Autodesk Inventor part; units mm, degrees
ref_plane "Arbeitsebene1" through (5, -117, 0) normal (0, 1, 0) x (1, 0, 0)
ref_plane "YZ Plane" through (0, 0, 0) normal (1, 0, 0) x (0, 1, 0)
ref_plane "XZ Plane" through (0, 0, 0) normal (0, 1, 0) x (-1, 0, 0)
sketch "Skizze1" plane through (0, 0, 0) normal (0, 0, 1) x (1, 0, 0)
  line L0 (0, 0) -> (60, 0)
  line L1 (60, 0) -> (60, -150)
  line L2 (60, -150) -> (0, -150)
  line L3 (0, -150) -> (0, 0)
  circle A0 centre (30, -117) radius 9
  dimension "d0" = 60
  dimension "d1" = 150
  dimension "d2" = 18
extrude "Extrusion1" add sketch "Skizze1" along normal blind 10
sketch "Skizze2" plane through (0, -150, 0) normal (0, -1, 0) x (1, 0, 0)
  point P0 (0, 0)
  point P1 (6.5, 5)
  point P2 (53.5, 5)
sketch "Skizze3" plane through (0, 0, 0) normal (0, 0, -1) x (-1, 0, 0)
  line L0 (-5, -117) -> (-55, -117)
  point P0 (0, 0)
ref_plane "Arbeitsebene1" through (5, -117, 0) normal (0, 1, 0) x (1, 0, 0)
split "Trennen1" plane through (5, -117, 0) removes the side toward (0, 1, 0)
hole "Bohrung2" at (6.5, -150, 5) at (53.5, -150, 5) direction (0, 1, 0) diameter 6.6 end through all
properties part number "Steher oben Rohr"
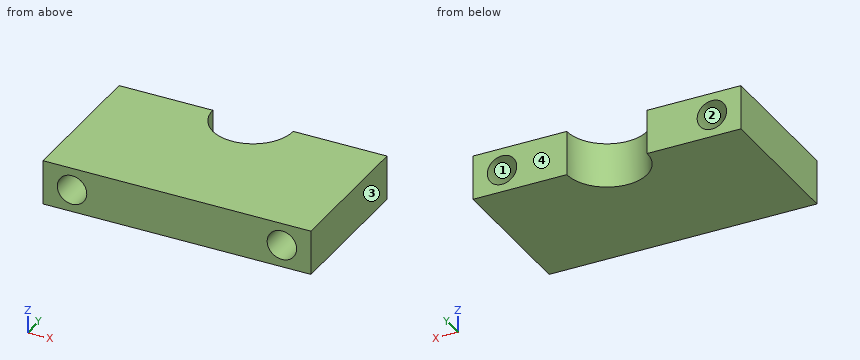
Can you work these out from the model? Positions are in its coordinate system, mm. Face numbers are marked on the shaded views. Round coordinates to 2 decimals unless told otherwise and drop trailing zeros. Loops run counter-clockwise (first coordinate to the right, second up) from the corner with the lowest first, then second, coordinate; pieces in that order, holes last. Notation, with made-up numbers: (-22, 78.5) - (-18, 78.5) arc R10 cw to (-18, 93.5) - close; hole circle Ø11 at (1.25, 13). An arc over 180 degrees is marked (long way). Write item = value, one per line. Start each with the question number.
(1) If we section it at B-B (x = 6.5): Please give me the cut outline in (y, z), and give its area (3 significant figures).
(2) If I drill on probe 1 along X at (y, z) = (-136.5, 5); probe 2 along Z at (x, y) = (6.5, -137.5); probe 3 along X at (y, z) = (-138.5, 2.75), over which ranges is the centre line in solid material (lowest first)? Write a range as [from, to].
(3) If we mould it in two halves opening along X, with no side actions, what happens to the marked faces 1, 2, 3 and 4? For each: released by +X, released by -X, zero draft, split by the parting line, or undercut.
(4) If we section it at D-D (y = -140.5): Please give me the cut outline in (x, z).
(5) If we section it at C-C (y = -125): Please give me the cut outline in (x, z), and give its area (3 significant figures).
(6) If we section it at A-A (z = 5): Please give me the cut outline in (x, y).
(7) For P1, Ø4, axis at x = 27.5, z = 9, coming from the +Y side; P2, Ø6, axis at x = 19, y = -145.5, coming from the -Z side; P3, Ø4, axis at x = 53.5, z = 5, coming from the +Y side, each with a flat end and sliding along its axis, tell me the tip position at first contact or that it passes through.
Ans:
q1.outline = (-150, 0) - (-117, 0) - (-117, 1.7) - (-150, 1.7) - close; (-150, 8.3) - (-117, 8.3) - (-117, 10) - (-150, 10) - close
q1.area = 112 mm²
q2.probe_1 = [0, 3.2], [9.8, 50.2], [56.8, 60]
q2.probe_2 = [0, 1.7], [8.3, 10]
q2.probe_3 = [0, 4.09], [8.91, 51.09], [55.91, 60]
q3.face_1 = undercut
q3.face_2 = undercut
q3.face_3 = released by +X
q3.face_4 = zero draft
q4.outline = (0, 0) - (60, 0) - (60, 10) - (0, 10) - close; hole circle Ø6.6 at (6.5, 5); hole circle Ø6.6 at (53.5, 5)
q5.outline = (0, 0) - (25.88, 0) - (25.88, 10) - (0, 10) - close; (34.12, 0) - (60, 0) - (60, 10) - (34.12, 10) - close; hole circle Ø6.6 at (6.5, 5); hole circle Ø6.6 at (53.5, 5)
q5.area = 449 mm²
q6.outline = (0, -150) - (3.2, -150) - (3.2, -117) - (0, -117) - close; (9.8, -150) - (50.2, -150) - (50.2, -117) - (39, -117) arc R9 cw to (21, -117) - (9.8, -117) - close; (56.8, -150) - (60, -150) - (60, -117) - (56.8, -117) - close
q7.P1 = -124.79
q7.P2 = 0
q7.P3 = through
